from build123d import *

# Parameters (mm, degrees)
SKETCH_1_W                      = 20
SKETCH_1_H                      = 8
EXTRUDE_1_DEPTH                 = 10
CUT_EXTRUDE_2_DEPTH             = 3
CUT_EXTRUDE_3_REACH             = 16.697
CUT_EXTRUDE_3_DIRECTION_2_REACH = 16.697
CUT_EXTRUDE_START               = 3.5
CUT_EXTRUDE_4_DEPTH             = 3.5
CUT_EXTRUDE_START_2             = -3.424924247
CUT_EXTRUDE_4_2_DEPTH           = 1.95709957
SKETCH_7_W                      = 19.5
SKETCH_7_H                      = 7.5
CUT_EXTRUDE_5_DEPTH             = 1
EXTRUDE_6_DEPTH                 = 0.1
MIRROR_2_COPY_1_DEPTH           = 0.1


with BuildPart() as part:
    # 草圖1 → 伸長1 (new body)
    with BuildSketch(Plane(origin=(0, 0, 0), x_dir=(1, 0, 0), z_dir=(0, 1, 0))):
        Rectangle(SKETCH_1_W, SKETCH_1_H)
    extrude(amount=EXTRUDE_1_DEPTH)

    # 草圖2 → 伸長2 (cut)
    with BuildSketch(Plane(origin=(0, 10, 0), x_dir=(1, 0, 0), z_dir=(0, 1, 0))):
        Polygon((-9.5, 0.5), (-9.5, -0.5), (0, -3.5), (9.5, -0.5), (9.5, 0.5), (0, 3.5), align=None)
    extrude(amount=-CUT_EXTRUDE_2_DEPTH, mode=Mode.SUBTRACT)

    # 伸長3: up to this plane
    cut_extrude_3_end = Plane(origin=(0, 7, -3.5), z_dir=(-0.3011313679370976, 0, -0.9535826651341416))
    # 草圖4 → 伸長3 (cut, up to the surface)
    with BuildSketch(Plane.XY, mode=Mode.PRIVATE) as cut_extrude_3_sk1:
        Polygon((0, 10), (-9.5, 10), (-9.5, 5.5), (0, 3.5), align=None)
    cut_extrude_3_tool1 = split(extrude(cut_extrude_3_sk1.sketch, amount=-CUT_EXTRUDE_3_REACH, mode=Mode.PRIVATE), bisect_by=cut_extrude_3_end, keep=Keep.BOTH, mode=Mode.PRIVATE)
    add(cut_extrude_3_tool1.solids().sort_by_distance((-4.462121, 7.219697, 0))[0], mode=Mode.SUBTRACT)

    # 伸長3 direction 2: up to this plane
    cut_extrude_3_direction_2_end = Plane(origin=(-9.5, 7, 0.5), z_dir=(-0.3011313679370972, 0, 0.9535826651341417))
    # 草圖4 → 伸長3 direction 2 (cut, up to the surface)
    with BuildSketch(Plane.XY, mode=Mode.PRIVATE) as cut_extrude_3_direction_2_sk1:
        Polygon((0, 10), (-9.5, 10), (-9.5, 5.5), (0, 3.5), align=None)
    cut_extrude_3_direction_2_tool1 = split(extrude(cut_extrude_3_direction_2_sk1.sketch, amount=CUT_EXTRUDE_3_DIRECTION_2_REACH, mode=Mode.PRIVATE), bisect_by=cut_extrude_3_direction_2_end, keep=Keep.BOTH, mode=Mode.PRIVATE)
    add(cut_extrude_3_direction_2_tool1.solids().sort_by_distance((-4.462121, 7.219697, 0))[0], mode=Mode.SUBTRACT)

    # 伸長4: read off the stored shape, not the designer's step
    # 伸長4 outline → 伸長4 (cut)
    with BuildSketch(Plane(origin=(0, 0, 0), x_dir=(1, 0, 0), z_dir=(0, 1, 0)).offset(CUT_EXTRUDE_START)):
        Polygon((9.5, -0.5), (9.5, 0.5), (0, 3.5), (0, -3.5), align=None)
    extrude(amount=CUT_EXTRUDE_4_DEPTH, mode=Mode.SUBTRACT)

    # Cut-Extrude 4 2 outline → Cut-Extrude 4 2 (add)
    with BuildSketch(Plane(origin=(0, 0, 0), x_dir=(0.978549784986749, 0.206010481049842, 0), z_dir=(0.206010481049842, -0.978549784986749, 0)).offset(CUT_EXTRUDE_START_2)):
        Polygon((0.721036684, 3.5), (0.721036684, -3.5), (10.429280603, -0.5), (10.429280603, 0.5), align=None)
    extrude(amount=CUT_EXTRUDE_4_2_DEPTH)

    # 草圖7 → 伸長5 (cut)
    with BuildSketch(Plane(origin=(0, 10, 0), x_dir=(1, 0, 0), z_dir=(0, 1, 0))):
        Rectangle(SKETCH_7_W, SKETCH_7_H)
    extrude(amount=-CUT_EXTRUDE_5_DEPTH, mode=Mode.SUBTRACT)

    # 草圖8 → 伸長6 (add)
    with BuildSketch(Plane(origin=(-1.005037783, 0, -3.182619647), x_dir=(0.9535826651341416, 0, -0.3011313679370976), z_dir=(0.3011313679370976, 0, 0.9535826651341416))):
        Polygon((-8.908469635, 5.5), (-8.908469635, 7.25), (-5.908469635, 7.25), (-5.908469635, 4.897737264), align=None)
    extrude_6 = extrude(amount=EXTRUDE_6_DEPTH)

    # 鏡射1: 伸長6 across plane
    add(extrude_6.mirror(Plane.XY))

    # 鏡射2: 伸長6 across plane
    add(extrude_6.mirror(Plane(origin=(0, 0, 0), x_dir=(0, 0, 1), z_dir=(1, 0, 0))))

    # 鏡射2 copy 1 sketch → 鏡射2 copy 1 (add)
    with BuildSketch(Plane(origin=(1.005037783, 0, 3.182619647), x_dir=(-0.9535826651341415, 0, 0.301131367937098), z_dir=(-0.301131367937098, 0, -0.9535826651341415))):
        Polygon((-8.908469635, 5.5), (-8.908469635, 7.25), (-5.908469635, 7.25), (-5.908469635, 4.897737264), align=None)
    extrude(amount=MIRROR_2_COPY_1_DEPTH)


solid = part.part
Verification items for the finished model (mm, model axes). A direction names the side the tool comes from. Coordinates: 2 decimals unless noted, no trailing zeros. Write each loop counter-clockwise with the first axis right and the second up, starting at its lowest first coordinate (ties: lowest second). Pieces come first, ordered by that corner, then holes. Notation, with made-up numbers: M 11,-23.75 L 15,-23.75 A16 cw 15,-18.75 Z; hole C -26.5,9.25 d5. An arc over 180 degrees is marked long. One line per question, with ' | ' between items.
1) Release check for a two-part mould opening along Z. For faces 1 (the face through (0, 5, -4)), 2 (the face through (-0.1, 9.5, 3.75)), 3 (the face through (-10, 5, 0)) record: +Z half, -Z half, draft (parallel to the pull), parting line (faces both ways), or undercut.
Solutions:
face 1: -Z half | face 2: undercut | face 3: draft
2) Sectioned sample at A-A on y = 7.75. Record the cut outline in (x, z), then the cut area to 3 significant figures.
Solutions:
outline: M -10,-4 L 10,-4 L 10,4 L -10,4 Z; hole M -9.5,-0.5 L 0,-3.5 L 9.5,-0.5 L 9.5,0.5 L 0,3.5 L -9.5,0.5 Z | area: 84.0 mm^2
3) Material ranges on L1, parallel to X at y = 8.5, z = 0.25; L2, parallel to Z at x = 1, y = 9.5; L3, parallel to Y at x = -7.25, z = 1.5, recorded low to high.
Solutions:
L1: -10 to -9.5, 9.5 to 10 | L2: -4 to -3.75, 3.75 to 4 | L3: 0 to 9
4) Depth check by flat-ended pin: pin 1 Ø2 at (x, z) = (6, 2) entering from +Y; pin 2 Ø0.5 at (x, z) = (-7.5, 0.5) entering from +Y; pin 3 Ø2 at (x, z) = (-3, 1) entering from +Y; pin 4 Ø4 at (x, z) = (1, 0.5) entering from -Y. Enter the tip coordinate at first touch or a pass-through.
Solutions:
pin 1: y = 9 | pin 2: y = 5.13 | pin 3: y = 4.34 | pin 4: y = 0
5) Sectioned sample at B-B on z = 2. Record the cut outline in (x, y), then the cut area to 3 significant figures.
Solutions:
outline: M -10,0 L 10,0 L 10,10 L 9.75,10 L 9.75,9 L 4.75,9 L 4.75,4.5 L 0,3.5 L -4.75,4.5 L -4.75,9 L -9.75,9 L -9.75,10 L -10,10 Z | area: 133 mm^2
6) Sectioned sample at D-D on y = 4.5. Record the cut outline in (x, z).
Solutions:
outline: M -10,-4 L 10,-4 L 10,4 L -10,4 Z; hole M -4.75,-2 L 0,-3.5 L 4.75,-2 L 4.75,2 L 0,3.5 L -4.75,2 Z
7) Sectioned sample at C-C on x = 2. Record the cut outline in (y, z).
Solutions:
outline: M 0,-4 L 10,-4 L 10,-3.75 L 9,-3.75 L 9,-2.87 L 3.92,-2.87 L 3.92,2.87 L 9,2.87 L 9,3.75 L 10,3.75 L 10,4 L 0,4 Z
8) Access from +Z, -Z, +X, -X, +Y, -Y to the whole of each face (thin tool, end or side, straight path). Record for faces 4 (the face through (0, 0, 0)), 5 (the face through (-8.019, 6.352, -0.863)).
Solutions:
face 4: +Z, -Z, +X, -X, -Y | face 5: +Y
